from build123d import *

# Parameters (mm, degrees)
SKETCH007_R              = 1.7
PAD019_DEPTH             = 13.5
FILLET006_R              = 1.5
SKETCH035_R              = 4
SKETCH035_R_2            = 1.7
PAD020_DEPTH             = 13.5
CLONE161_PLACEMENT_ANGLE = 180


with BuildPart() as part:
    # Sketch007 → Pad019 (new body)
    with BuildSketch(Plane(origin=(0, 19.25, 0), x_dir=(-1, 0, 0), z_dir=(0, 1, 0))):
        with BuildLine():
            ThreePointArc((12, 26), (8, 22), (12, 18))
            Line((12, 18), (37.984377, 18))
            ThreePointArc((38.844741, 17.728728), (38.435435, 17.930575), (37.984377, 18))
            Line((38.844741, 17.728728), (51.705713, 8.723378))
            ThreePointArc((51.705713, 8.723378), (57.276616, 9.705705), (56.294304, 15.27661))
            Line((43.045936, 24.553216), (56.294304, 15.27661))
            ThreePointArc((43.045936, 24.553216), (40.862971, 25.629736), (38.457325, 26))
            Line((12, 26), (38.457325, 26))
        make_face()
        with Locations((12, 22)):
            Circle(SKETCH007_R, mode=Mode.SUBTRACT)
        with Locations((54, 12)):
            Circle(SKETCH007_R, mode=Mode.SUBTRACT)
    extrude(amount=PAD019_DEPTH)

    # Fillet006
    fillet006_edges = [part.edges().sort_by_distance(p)[0] for p in [
        (-49.67012, 32.75, 19.914913),
        (-49.67012, 19.25, 19.914913),
    ]]
    fillet(fillet006_edges, radius=FILLET006_R)

    # Sketch035 (on Face12 of Fillet006) → Pad020 (join)
    with BuildSketch(Plane(origin=(0, 32.75, 0), x_dir=(-1, 0, 0), z_dir=(0, 1, 0))):
        with Locations((54, 12)):
            Circle(SKETCH035_R)
        with Locations((54, 12)):
            Circle(SKETCH035_R_2, mode=Mode.SUBTRACT)
        with Locations((12, 22)):
            Circle(SKETCH035_R)
        with Locations((12, 22)):
            Circle(SKETCH035_R_2, mode=Mode.SUBTRACT)
    extrude(amount=-PAD020_DEPTH)


with BuildPart() as part_1:
    # Body002 placement: moved
    add(part.part.moved(Location((0, -5, 0))))


with BuildPart() as part_2:
    # Clone161 placement: moved
    add(part_1.part.moved(Location((47, 47, 8))).rotate(Axis((47, 47, 8), (0, 0, 1)), CLONE161_PLACEMENT_ANGLE))


solid = part_2.part
Can you work these out from the model? Positions are in its coordinate system, mm. A direction names the side the tool comes from. Give positions to 0.01 mm unless a question says otherwise; leave off trailing zeros. Loops run counter-clockwise (first coordinate to the right, second up) from the corner with the lowest first, then second, coordinate; pieces in that order, holes last. Notation, with made-up numbers: (65, 73) - (82, 73) arc R13 ccw to (82, 86) - close; hole circle Ø6 at (30.25, 51). An arc over 180 degrees is marked (long way). Return JSON: item names as keys, results as strings.
1. I want a section at A-A on y = 22.5. Please give me the cut outline in (x, z), and give its area (3 significant figures).
Output values:
{"outline": "(59, 26) - (84.98, 26) arc R1.5 cw to (85.84, 25.73) - (98.71, 16.72) arc R4 ccw to (103.29, 23.28) - (90.05, 32.55) arc R8 ccw to (85.46, 34) - (59, 34) arc R4 ccw to start; hole circle Ø3.4 at (59, 30); hole circle Ø3.4 at (101, 20)", "area": "393 mm²"}
2. If I drill on line 1 (Z direction, x = 60, y = 21); line 2 (Z direction, x = 101, y = 26.5); line 3 (X direction, y = 28.5, z = 30.5), over which ranges is the centre line in solid material (lowest first)?
Output values:
{"line 1": "z = 26 to 28.63, 31.37 to 34", "line 2": "z = 16 to 18.3, 21.7 to 24.88", "line 3": "x = 55.03 to 57.38, 60.62 to 92.98"}
3. I'm going to push flat-ended pins straight in: pin 1 Ø6 at (x, y) = (93.5, 26) entering from -Z; pin 2 Ø1 at (y, z) = (21.5, 26) entering from +X; pin 3 Ø5 at (y, z) = (24, 19) entering from -X; pin 4 Ø2 at (x, z) = (100, 28) entering from +Y. Where does each tip first touch, or does it pass through?
Output values:
{"pin 1": "stops at z = 18.27", "pin 2": "stops at x = 100.12", "pin 3": "stops at x = 91.88", "pin 4": "passes through"}
4. We'd pull the mould along X, two halves only. Please class faces 1 (the face through (99.3, 26.09, 20.07)), 2 (the face through (72.41, 19.7, 33.57)), 3 (the face through (92.185, 26.074, 21.289)): +X half, -X half, draft (parallel to the pull), parting line (faces both ways), or undercut.
Output values:
{"face 1": "undercut", "face 2": "draft", "face 3": "-X half"}
5. For faces 4 (the face through (72, 26, 26)), 5 (the face through (71.81, 19.7, 26.43)), 6 (the face through (71.81, 32.3, 26.43)), 7 (the face through (72.41, 32.3, 33.57)), 8 (the face through (57.3, 26.09, 30.07)), which set-ups out of +Z, -Z, +X, -X, +Y, -Y let a thin tool reach every point of the face, with its end or its side?
Output values:
{"face 4": "-Z, -X, +Y, -Y", "face 5": "-Z, -Y", "face 6": "-Z, +Y", "face 7": "+Z, +X, +Y", "face 8": "+Y, -Y"}
